from build123d import *

# Parameters (mm, degrees)
AUFSATZ_LINEAR_AUSTRAGEN1_DEPTH                     = 55
SCHNITT_LINEAR_AUSTRAGEN1_DEPTH                     = 183.25960194184557
SCHNITT_LINEAR_AUSTRAGEN2_DEPTH                     = 215.5675884191273
STIRNSENKUNG_F_R_M4_SENKSCHRAUBE_KOPF_B_D           = 4.5
STIRNSENKUNG_F_R_M4_SENKSCHRAUBE_KOPF_B_CBORE_D     = 8.6
STIRNSENKUNG_F_R_M4_SENKSCHRAUBE_KOPF_B_CBORE_DEPTH = 50


with BuildPart() as part:
    # Skizze2 → Aufsatz-Linear austragen1 (new body)
    with BuildSketch(Plane.XY):
        Polygon((97.25, -71.99999999999999), (-97.25, -72.00000000000001), (-97.25, 72), (97.25, 72.00000000000001), align=None)
    extrude(amount=AUFSATZ_LINEAR_AUSTRAGEN1_DEPTH)

    # Skizze3 → Schnitt-Linear austragen1 (cut, through all)
    with BuildSketch(Plane.XZ.offset(72)):
        with BuildLine():
            Line((-47.250000000000014, 54.99999999999999), (-31.187648825052438, 55))
            Line((-31.187648825052438, 55), (-49.06524576519668, 93.49392426446363))
            Line((-49.06524576519668, 93.49392426446363), (-152.6979191152644, 34.404714288264984))
            Line((-152.6979191152644, 34.404714288264984), (-97.25000000000001, -29.09207494836323))
            Line((-97.25000000000001, -29.09207494836323), (-97.25, 4.99999999999999))
            ThreePointArc((-97.25, 4.99999999999999), (-82.60533905932738, 40.35533905932737), (-47.250000000000014, 54.99999999999999))
        make_face()
    schnitt_linear_austragen1 = extrude(amount=-SCHNITT_LINEAR_AUSTRAGEN1_DEPTH, mode=Mode.SUBTRACT)

    # Spiegeln3: Schnitt-Linear austragen1 across plane
    add(schnitt_linear_austragen1.mirror(Plane(origin=(0, 0, 0), x_dir=(0, 0, 1), z_dir=(1, 0, 0))), mode=Mode.SUBTRACT)

    # Skizze6 → Schnitt-Linear austragen2 (cut, through all)
    with BuildSketch(Plane(origin=(97.25, 0, 0), x_dir=(0, 0, -1), z_dir=(1, 0, 0))):
        with BuildLine():
            Line((-4.999999999999997, 72.00000000000001), (11.062351174947562, 72.00000000000003))
            Line((11.062351174947562, 72.00000000000003), (-41.4687477452512, 93.52582627901205))
            Line((-41.4687477452512, 93.52582627901205), (-130.24502976788665, 42.907423802585875))
            Line((-130.24502976788665, 42.907423802585875), (-54.99999999999999, -43.260242586178926))
            Line((-54.99999999999999, -43.260242586178926), (-55, 22))
            ThreePointArc((-55, 22), (-40.35533905932737, 57.35533905932739), (-4.999999999999997, 72.00000000000001))
        make_face()
    schnitt_linear_austragen2 = extrude(amount=-SCHNITT_LINEAR_AUSTRAGEN2_DEPTH, mode=Mode.SUBTRACT)

    # Spiegeln4: Schnitt-Linear austragen2 across plane
    add(schnitt_linear_austragen2.mirror(Plane.ZX), mode=Mode.SUBTRACT)

    # Stirnsenkung für M4 Senkschraube (Kopf Button)1 (through all)
    with Locations(Plane.XY.offset(55)):
        with Locations((-42.25, 7)):
            stirnsenkung_f_r_m4_senkschraube_kopf_b = CounterBoreHole(STIRNSENKUNG_F_R_M4_SENKSCHRAUBE_KOPF_B_D / 2, STIRNSENKUNG_F_R_M4_SENKSCHRAUBE_KOPF_B_CBORE_D / 2, STIRNSENKUNG_F_R_M4_SENKSCHRAUBE_KOPF_B_CBORE_DEPTH)

    # Spiegeln5: Stirnsenkung für M4 Senkschraube (Kopf Button)1 across plane
    add(stirnsenkung_f_r_m4_senkschraube_kopf_b.mirror(Plane(origin=(0, 0, 0), x_dir=(0, 0, 1), z_dir=(1, 0, 0))), mode=Mode.SUBTRACT)


solid = part.part
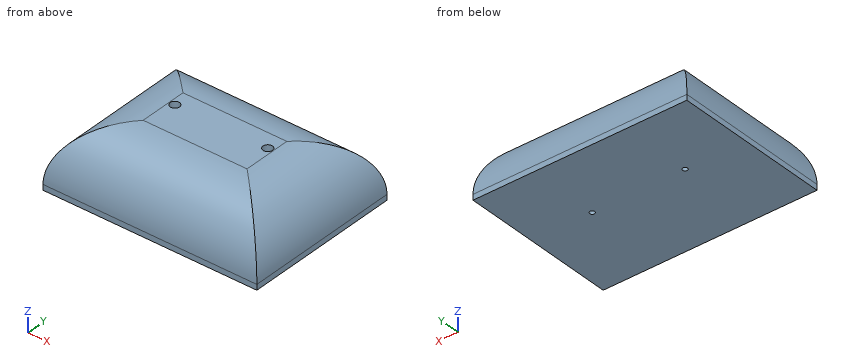
Source: CAD feature listing. Evaluate the final solid. Frame: model axes, mm. Give positions to 0.01 mm unless a question says otherwise; leave off trailing zeros. Write each loop counter-clockwise with the first axis right and the second up, starting at its lowest first coordinate (ties: lowest second). Pieces come first, ordered by that corner, then holes. Notation, with made-up numbers: M -19,9 L 4,9 A25 cw 4,36 Z; hole C -16,44.5 d6. An arc over 180 degrees is marked long. Answer as a JSON object with one key per item and string values.
Q1. Cut plane C-C, the plane z = 43. Return the cut outline in (x, y), then the cut area to 3 significant figures.
Geometry check:
{"outline": "M -79.75,-54.5 L 79.75,-54.5 L 79.75,54.5 L -79.75,54.5 Z; hole C -42.25,7 d8.6; hole C 42.25,7 d8.6", "area": "17,300 mm^2"}
Q2. Contact query for flat-ended pins moving along their axis: P1, Ø5, axis at x = -34, y = 23.5, coming from the -Z side; P2, Ø1.5, axis at x = -27, y = -46.5, coming from the +Z side; P3, Ø10, axis at x = -31, z = 42.5, coming from the -Y side; P4, Ø6, axis at x = -63.5, z = 26, coming from the -Y side. Output: stop coordinate, or through.
Geometry check:
{"P1": "stops at z = 0", "P2": "stops at z = 49", "P3": "stops at y = -60", "P4": "stops at y = -68.65"}
Q3. Cut plane B-B, the plane x = 42.25. Return the cut outline in (y, z).
Geometry check:
{"outline": "M -72,0 L 4.75,0 L 4.75,5 L 2.7,5 L 2.7,55 L -22,55 A50 ccw -72,5 Z; M 9.25,0 L 72,0 L 72,5 A50 ccw 22,55 L 11.3,55 L 11.3,5 L 9.25,5 Z"}
Q4. Cut plane A-A, the plane y = 7. Return the cut outline in (x, z), then the cut area to 3 significant figures.
Geometry check:
{"outline": "M -97.25,0 L -44.5,0 L -44.5,5 L -46.55,5 L -46.55,55 L -47.25,55 A50 ccw -97.25,5 Z; M -40,0 L 40,0 L 40,5 L 37.95,5 L 37.95,55 L -37.95,55 L -37.95,5 L -40,5 Z; M 44.5,0 L 97.25,0 L 97.25,5 A50 ccw 47.25,55 L 46.55,55 L 46.55,5 L 44.5,5 Z", "area": "8,720 mm^2"}
Q5. Cut plane D-D, the plane x = -20.5. Return the cut outline in (y, z).
Geometry check:
{"outline": "M -72,0 L 72,0 L 72,5 A50 ccw 22,55 L -22,55 A50 ccw -72,5 Z"}
Q6. Ray query, line 1 along X through (y, z) = (4, 15); line 2 along X through (y, z) = (9, 45); line 3 along Y through (x, z) = (42.25, 1.9). Return the intervals inside material, ascending.
Geometry check:
{"line 1": "x = -96.24 to -45.33, -39.17 to 39.17, 45.33 to 96.24", "line 2": "x = -77.25 to -46.06, -38.44 to 38.44, 46.06 to 77.25", "line 3": "y = -72 to 4.75, 9.25 to 72"}
